Could you check a few things on this model? Use its own coordinates, in mm. A direction names the side the tool comes from. Give positions to 0.01 mm unless a question says otherwise; leave off trailing zeros. Order: outer loops, then holes, each group sorted by start corner. A loop starts at its lowest first (then second) coordinate and runs counter-clockwise, first axis right, second up. Notation, with made-up numbers: (-26, 62) - (21, 62) arc R16 ccw to (21, 89) - close; hole circle Ø11 at (-7, 6). An arc over 180 degrees is marked (long way). One line per question, with ' | ' between items. Start each with the question number.
1. Imagine slicing it at B-B (z = -9). Please give me the cut outline in (x, y) (1 decimal), and give its area (3 significant figures).
2. Imagine slicing it at C-C (x = 1). Please give me the cut outline in (y, z) (3 decimals).
3. I need wall thicknesses on probe 1 along Z at (x, y) = (-0.5, -1.5); probe 2 along Y at (x, z) = (0, 5.5) (1 decimal); probe 3 along Y at (x, z) = (4, -8.5) (3 decimals). Which ranges of each line are inside material? Lowest first, please. Write a range as from..to.
4. If we mould it in two halves opening along X, with no side actions, what happens to faces 1 (the cylindrical face through (-0.55, 0.43, 3.69)), 2 (the flat face through (7.048, 1, -4)), 3 (the flat face through (0, -1, 0)), 4 (the cylindrical face through (-1.57, -1.08, -11.57))? For each: released by +X, released by -X, zero draft, split by the parting line, or undercut.
5. For P1, Ø2.5, axis at x = 6, z = -5, coming from the -Y side, with a flat end and sliding along its axis, tell me the tip position at first contact or that it passes through.
6. Imagine slicing it at A-A (y = -1.65). Please give me the cut outline in (x, z), and give its area (3 significant figures).
7. Which directions (+Z, -Z, +X, -X, +Y, -Y) give clear straight access to the entire face, cutting with the end or side of a thin tool? Please do faces 5 (the flat face through (5, 0, -4)), 6 (the cylindrical face through (0.55, 0.43, -11.57)), 7 (the flat face through (-1, 0, -7.874)).
Autodesk Inventor part; units mm, degrees
ref_plane "YZ Plane" through (0, 0, 0) normal (1, 0, 0) x (0, 1, 0)
ref_plane "XZ Plane" through (0, 0, 0) normal (0, 1, 0) x (-1, 0, 0)
ref_plane "XY Plane" through (0, 0, 0) normal (0, 0, 1) x (1, 0, 0)
sketch "Sketch1" plane through (0, 0, 0) normal (0, 0, 1) x (1, 0, 0)
  circle A0 centre (0, 0) radius 0.6985
  circle A1 centre (0, 0) radius 1.905
  line L0 (0.6985, 0) -> (7.0485, 0)
  line L1 (7.0485, 0) -> (7.0485, 1.905)
  line L2 (7.0485, 1.905) -> (0.6985, 1.905)
  line L3 (0.6985, 1.905) -> (0.6985, 0)
  point P0 (0.6985, 1.7723)
  point P1 (1.905, 0)
  dimension "d0" = 1.397
  dimension "d1" = 3.81
  dimension "d4" = 6.35
  dimension "d5" = 1.905
extrude "Extrusion1" add sketch "Sketch1" along normal blind 7.493
fillet "Fillet1" radius 3.175 1 edges at (0.6985, 1.7723, 3.7465)
fillet "Fillet2" radius 0.5292 1 edges at (1.905, 0, 3.7465)
sketch "Sketch2" plane through (0, 0, 0) normal (0, 0, -1) x (-1, 0, 0)
  arc A0 (-0.6985, 1.905) -> (-0.1463, 1.8994) centre (-0.3902, 5.065) ccw
  line L0 (-7.0485, 1.905) -> (-0.6985, 1.905)
  line L1 (-7.0485, 0) -> (-7.0485, 1.905)
  line L2 (-2.376, 0) -> (-7.0485, 0)
  arc A1 (-1.8594, -0.4141) -> (-2.376, 0) centre (-2.376, -0.5292) ccw
  arc A2 (-1.8594, -0.4141) -> (-0.1463, 1.8994) centre (0, 0) ccw
  circle A3 centre (0, 0) radius 0.6985
  circle A4 centre (0, 0) radius 1.905
  circle A5 centre (0, 0) radius 2.032
  line L3 (-0.5019, 1.969) -> (-0.5019, 1.892)
  point P0 (-2.0278, -0.1307)
  point P1 (0.0205, 1.3968)
  point P2 (-0.7071, 1.905)
  dimension "d8" = 0.127
extrude "Extrusion2" add sketch "Sketch2" along normal blind 7.874 contours A5 A1 L2 L1 L0
extrude "Extrusion3" add sketch "Sketch2" along normal blind 7.493 from surface at 7.874 contours A0 A4 A1 A5 L0 | A5 A1 L2 L1 L0 | A2 A4
properties part number "outerhinge"
Results found:
1) outline: (0.1, 1.9) arc R1.9 ccw (long way) to (1.9, -0.4) arc R0.5 cw to (2.4, 0) - (7, 0) - (7, 1.9) - (0.7, 1.9) arc R3.2 cw to start; hole circle Ø1.4 at (0, 0) | area: 20.5 mm2
2) outline: (-1.621, -15.367) - (1.905, -15.367) - (1.905, 7.493) - (-1.621, 7.493) - (-1.621, 0) - (1.769, 0) - (1.769, -7.874) - (-1.621, -7.874) - close
3) probe 1: z = -15.37..-7.87, 0..7.49 | probe 2: y = -1.9..-0.7, 0.7..1.9 | probe 3: y = 0..1.905
4) face 1: undercut | face 2: released by +X | face 3: zero draft | face 4: split by the parting line
5) P1: stops at y = 0
6) outline: (-0.95, -15.37) - (0.95, -15.37) - (0.95, -7.87) - (-0.95, -7.87) - close; (-0.95, 0) - (0.95, 0) - (0.95, 7.49) - (-0.95, 7.49) - close | area: 28.5 mm2
7) face 5: +Z, -Z, +X, -Y | face 6: +Z, -Z | face 7: -X, -Y
